For this review, use the dimensioned drawing (mm, ordinates from the lowest corner) and the shaded views. Round coordinates to 2 decimals unless told otherwise and drop trailing zeros. Order: outer loops, then holes, each group sorted by start corner. A loop starts at its lowest first (then second) coordinate and runs counter-clockwise, first axis right, second up. Notation, with made-up numbers: M -22,-3 L -2,-3 A20 ccw -2,26 Z; hole C 28.25,-9.75 d10. An arc over 180 degrees is marked long. Answer as CSV lines item,"result". Start each with the question number.
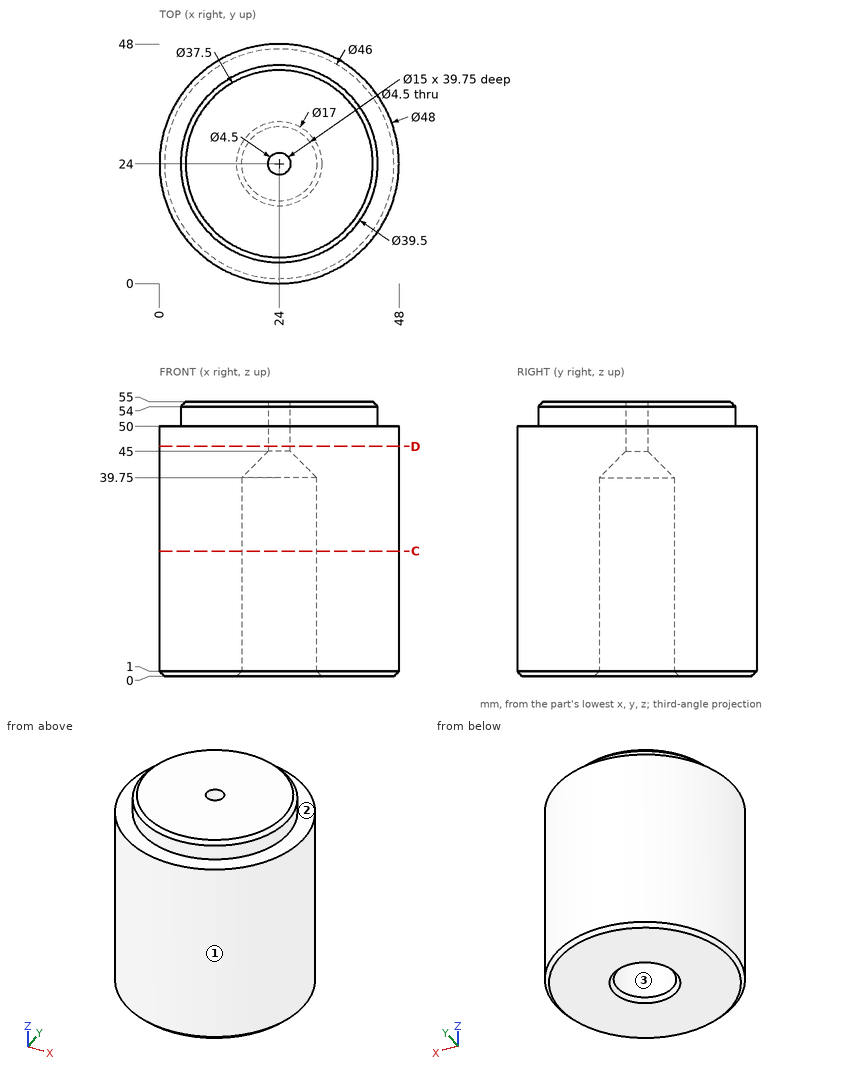
Item 1: The part is to be moulded in two halves that separate along X. For the marked faces 1, 2 and 3, say which applies: +X half, -X half, draft (parallel to the pull), parting line (faces both ways), or undercut.
Item 2: Consider section C-C (z = 25). State the section outline as (x, y) points, and give its area (3 significant figures).
Item 3: For pin 1 (2 mm diameter, centred on x = 16, z = 23, fed in from -Y); pin 2 (10 mm diameter, centred on y = 16.5, z = 40, fed in from -X); pin 3 (3 mm diameter, centred on x = 27, z = 46.5, fed in from -Y); pin 4 (2.5 mm diameter, centred on x = 24, y = 23.5, fed in from -Z), all flat-tipped, find the tip position at first contact; note any pin that passes through.
Item 4: Wall thickness on probe 1 along Y at (x, z) = (24, 21.5); probe 2 along X at (y, z) = (39, 48) (3 decimals); probe 3 along Y at (x, z) = (24, 51.25): over which ranges is each line inside the solid? List them lowest first. Write a range as [from, to].
Item 5: Consider section D-D (z = 46). State the section outline as (x, y) points.
Reported:
1,face 1,"parting line"
1,face 2,"draft"
1,face 3,"undercut"
2,outline,"C 24,24 d48; hole C 24,24 d15"
2,area,"1,630 mm²"
3,pin 1,"stops at y = 1.04"
3,pin 2,"stops at x = 0.13"
3,pin 3,"stops at y = 0.05"
3,pin 4,"passes through"
4,probe 1,"y = [0, 16.5], [31.5, 48]"
4,probe 2,"x = [5.265, 42.735]"
4,probe 3,"y = [4.25, 21.75], [26.25, 43.75]"
5,outline,"C 24,24 d48; hole C 24,24 d4.5"
